Autodesk Inventor part; units mm, degrees
ref_plane "YZ Plane" through (0, 0, 0) normal (1, 0, 0) x (0, 1, 0)
ref_plane "XZ Plane" through (0, 0, 0) normal (0, 1, 0) x (-1, 0, 0)
ref_plane "XY Plane" through (0, 0, 0) normal (0, 0, 1) x (1, 0, 0)
sketch "Sketch1" plane through (0, 0, 0) normal (0, 0, 1) x (1, 0, 0)
  line L0 (0, 0) -> (127, 0)
  line L1 (127, 0) -> (127, 53.975)
  line L2 (127, 53.975) -> (0, 53.975)
  line L3 (0, 53.975) -> (0, 0)
  line L4 (12.7, 53.975) -> (114.3, 53.975)
  line L5 (114.3, 53.975) -> (114.3, 74.295)
  line L6 (114.3, 74.295) -> (12.7, 74.295)
  line L7 (12.7, 74.295) -> (12.7, 53.975)
  circle A0 centre (27.94, 66.675) radius 3.0988
  circle A1 centre (63.5, 66.675) radius 3.0988
  circle A2 centre (99.06, 66.675) radius 3.0988
  dimension "d0" = 127
  dimension "d1" = 53.975
  dimension "d2" = 101.6
  dimension "d3" = 12.7
  dimension "d4" = 20.32
  dimension "d5" = 6.1976
  dimension "d6" = 35.56
  dimension "d12" = 12.7
  dimension "d13" = 12.7
  dimension "d14" = 50.8
  dimension "d15" = 12.7
  dimension "d16" = 35.56
extrude "Extrusion1" add sketch "Sketch1" along normal blind 4.7625
equation "\"d3\" = -0.5 * d2 + 0.5 * d0"
equation "\"d13\" = d12"
equation "\"d14\" = 0.5 * d2"
equation "\"d15\" = d13"
equation "\"d16\" = d6"
properties part number "Top"
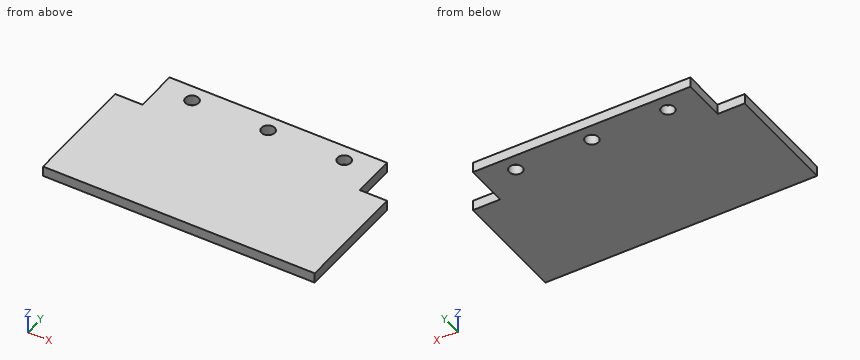
The listing builds one solid part. Answer for the finished solid, in the listing's coordinates (mm). Give positions to 0.01 mm unless a question says otherwise; leave off trailing zeros. Write each loop counter-clockwise with the first axis right and the second up, starting at its lowest first coordinate (ties: lowest second). Pieces come first, ordered by that corner, then holes. Notation, with made-up numbers: (41.25, -14.5) -> (67.25, -14.5) arc R15 cw to (67.25, 8.5) -> close; hole circle Ø4 at (-9.5, 21). An arc over 180 degrees is marked (long way). Use one line per item in the form item = value.
1) Straight lines are drawn through the part: probe 1 along Y at (x, z) = (99.06, 1.9) (3 decimals); probe 2 along X at (y, z) = (64, 2.4); probe 3 along X at (y, z) = (68.5, 3.65). For each, find the intervals that lie inside material, in ascending order.
Result:
probe_1 = 0 to 63.576, 69.774 to 74.295
probe_2 = 12.7 to 26.38, 29.5 to 61.94, 65.06 to 97.5, 100.62 to 114.3
probe_3 = 12.7 to 25.44, 30.44 to 61, 66 to 96.56, 101.56 to 114.3
2) Section A-A on x = 63.5 is taken. Write down the section's boundary in (y, z) (1 decimal), plus the area to 3 significant figures.
Result:
outline = (0, 0) -> (63.6, 0) -> (63.6, 4.8) -> (0, 4.8) -> close; (69.8, 0) -> (74.3, 0) -> (74.3, 4.8) -> (69.8, 4.8) -> close
area = 324 mm²
3) Each of these flat-tipped pins is pushed along its axis until it touches: P1, Ø1.4, axis at x = 8.5, z = 2.5, coming from the +Y side (3 decimals); P2, Ø1.4, axis at y = 68, z = 3, coming from the -X side. Where does it stop, or does it pass through?
Result:
P1 = 53.975
P2 = 12.7
4) Section B-B on z = 3.75 is taken. Write down the section's boundary in (x, y) (3 decimals), plus the area to 3 significant figures.
Result:
outline = (0, 0) -> (127, 0) -> (127, 53.975) -> (114.3, 53.975) -> (114.3, 74.295) -> (12.7, 74.295) -> (12.7, 53.975) -> (0, 53.975) -> close; hole circle Ø6.198 at (27.94, 66.675); hole circle Ø6.198 at (63.5, 66.675); hole circle Ø6.198 at (99.06, 66.675)
area = 8,830 mm²
